Part model, mm, in its own coordinate system. Give positions to 0.01 mm unless a question says otherwise; leave off trailing zeros. Order: outer loops, then holes, each group sorted by start corner. A loop starts at its lowest first (then second) coordinate and runs counter-clockwise, first axis right, second up. Notation, with made-up numbers: M 46,45.25 L 103,45.25 A20 ccw 103,78.25 Z; hole C -8.75,66 d6. An arc over 180 degrees is marked long. One line per question, with ' | ' between items.
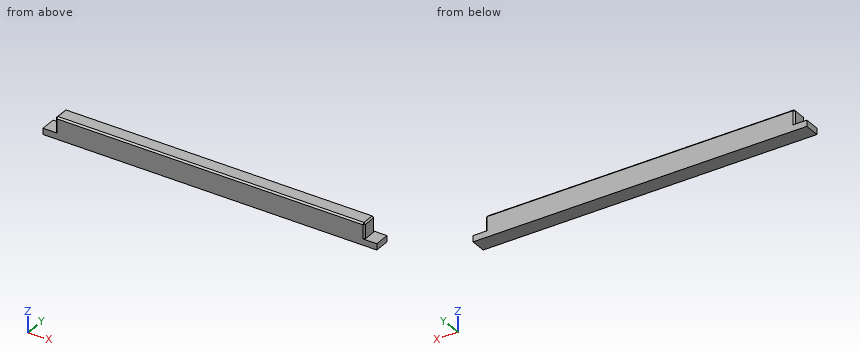
```python
from build123d import *

# Parameters (mm, degrees)
F0_W     = 100
F0_H     = 5
F1_DEPTH = 5
F0_W_2   = 4
F2_DEPTH = 2
F3_SIZE  = 0.5


with BuildPart() as f1:
    # F0 (on Top) → F1 (new body)
    with BuildSketch(Plane.XY):
        with Locations((3.835353, 2.5)):
            Rectangle(F0_W, F0_H)
    extrude(amount=F1_DEPTH)

    # F0 (on Top) → F2 (join)
    with BuildSketch(Plane.XY):
        with Locations((-48.164647, 2.5)):
            Rectangle(F0_W_2, F0_H)
        with Locations((3.835353, 2.5)):
            Rectangle(F0_W, F0_H)
        with Locations((55.835353, 2.5)):
            Rectangle(F0_W_2, F0_H)
    extrude(amount=-F2_DEPTH)

    # F3
    f3_edges = [f1.edges().sort_by_distance(p)[0] for p in [
        (-46.164647, 2.5, 5),
        (3.835353, 0, 5),
        (53.835353, 2.5, 5),
        (3.835353, 5, 5),
        (53.835353, 5, 2.5),
        (53.835353, 0, 2.5),
        (-46.164647, 0, 2.5),
        (-46.164647, 5, 2.5),
    ]]
    chamfer(f3_edges, length=F3_SIZE)


solid = f1.part
```
1. Probe L1, parallel to X at y = 3.45, z = 1; L2, parallel to X at y = 1.8, z = 4.75. List the from-to ranges inside material, lowest first. Write a range as from..to.
Worked out:
L1: x = -46.16..53.84 | L2: x = -45.91..53.59
2. Drop flat-ended pins along their axis: pin 1 (2 mm diameter, centred on y = 3, z = 3, fed in from +X); pin 2 (1.3 mm diameter, centred on x = 56, y = 2, fed in from +Z). Give the stop position or say it passes through.
Worked out:
pin 1: stops at x = 53.84 | pin 2: stops at z = 0
3. Slice it at B-B on z = 3. Give the cut face in (x, y), then the cut area to 4 significant figures.
Worked out:
outline: M -46.16,0.5 L -45.66,0 L 53.34,0 L 53.84,0.5 L 53.84,4.5 L 53.34,5 L -45.66,5 L -46.16,4.5 Z | area: 499.5 mm2
4. Slice it at A-A on y = 3.05. Give the cut face in (x, z).
Worked out:
outline: M -50.16,-2 L 57.84,-2 L 57.84,0 L 53.84,0 L 53.84,4.5 L 53.34,5 L -45.66,5 L -46.16,4.5 L -46.16,0 L -50.16,0 Z
